Check sheet for the drawn part. Datum: minimum x, y, z corner. Units: mm. A direction names the side the tool comes from. Coordinates: 2 decimals unless noted, no trailing zeros. Write each loop counter-clockwise with the first axis right and the second up, starting at its lowest first coordinate (ties: lowest second). Pieces come first, ordered by that corner, then holes. Notation, with made-up numbers: (68, 59.5) -> (125, 59.5) arc R22 cw to (125, 77.5) -> close; hole circle Ø7 at (-38, 53.25). An arc over 180 degrees is marked (long way). Answer in a Markdown table with one row per item. Add a question column.
1. Depth check by flat-ended pin: P1, Ø1, axis at x = 142.5, y = 390.5, coming from the +Z side; P2, Ø12, axis at x = 231, z = 202, coming from the +Y side; P3, Ø8, axis at y = 493.5, z = 267, coming from the +X side. Enter the tip coordinate at first touch or a pass-through.
2. Scan lines: L1, parallel to Z at x = 96, y = 476; L2, parallel to X at y = 505, z = 355.5; L3, parallel to Y at x = 501, z = 146. Record each from-to range of solid material in increasing order. Write a range as from..to.
3. Cross-section at C-C on z = 253. Record the cut outline in (x, y).
4. Cross-section at D-D on x = 444. Record the cut outline in (y, z), and give its area (3 significant figures).
5. Cross-section at A-A on x = 84.5. Record the cut outline in (y, z), and give its area (3 significant figures).
6. Cross-section at B-B on y = 63. Record the cut outline in (x, z).
7. Set-up check for the marked faces 1, 2, 3 and 4: record each of +Z, -Z, +X, -X, +Y, -Y from which the full face is reachable in a straight line by a thin tool's end or side.
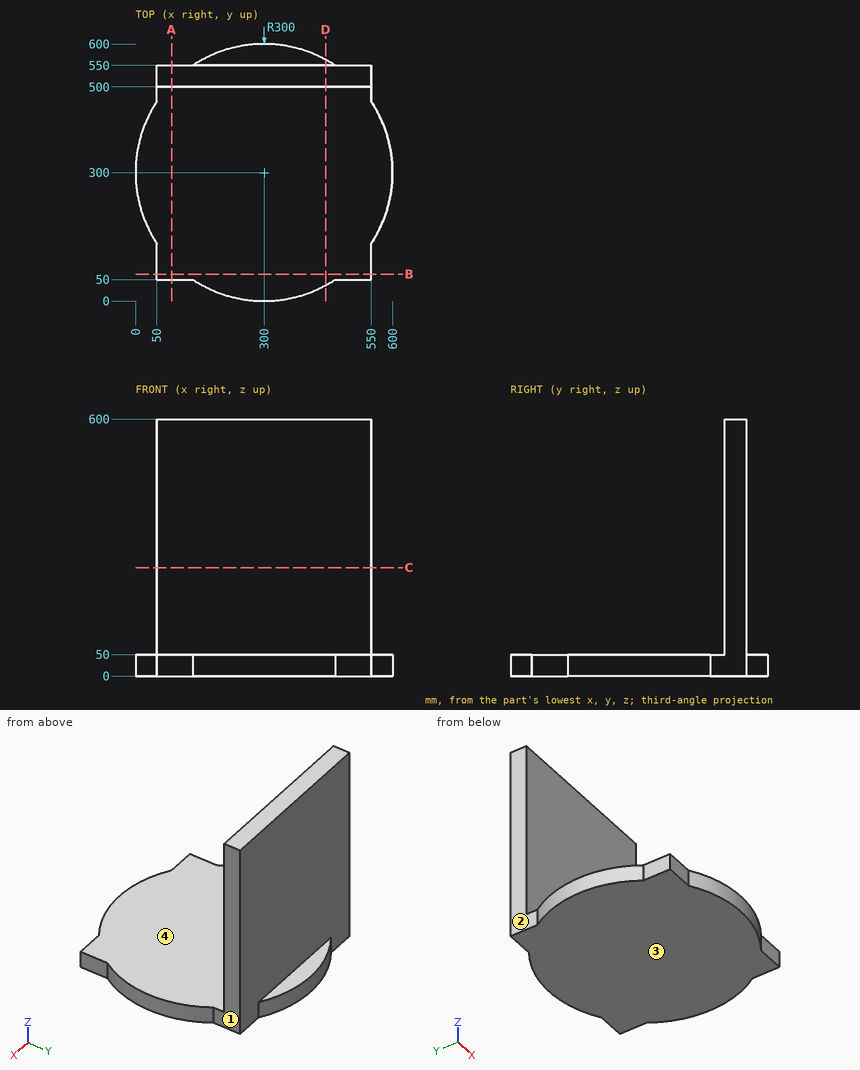
Results found:
| question | item | result |
|---|---|---|
| 1 | P1 | stops at z = 50 |
| 1 | P2 | stops at y = 550 |
| 1 | P3 | passes through |
| 2 | L1 | z = 0..50 |
| 2 | L2 | x = 50..550 |
| 2 | L3 | y = 500..550 |
| 3 | outline | (50, 500) -> (550, 500) -> (550, 550) -> (50, 550) -> close |
| 4 | outline | (36.82, 0) -> (563.18, 0) -> (563.18, 50) -> (550, 50) -> (550, 600) -> (500, 600) -> (500, 50) -> (36.82, 50) -> close |
| 4 | area | 53,800 mm^2 |
| 5 | outline | (50, 0) -> (550, 0) -> (550, 600) -> (500, 600) -> (500, 50) -> (50, 50) -> close |
| 5 | area | 52,500 mm^2 |
| 6 | outline | (50, 0) -> (550, 0) -> (550, 50) -> (50, 50) -> close |
| 7 | face 1 | +Z, -Z, +X, +Y |
| 7 | face 2 | +Z, -Z, -X, +Y |
| 7 | face 3 | -Z, +X, -X, +Y, -Y |
| 7 | face 4 | +Z, +X, -X, -Y |
